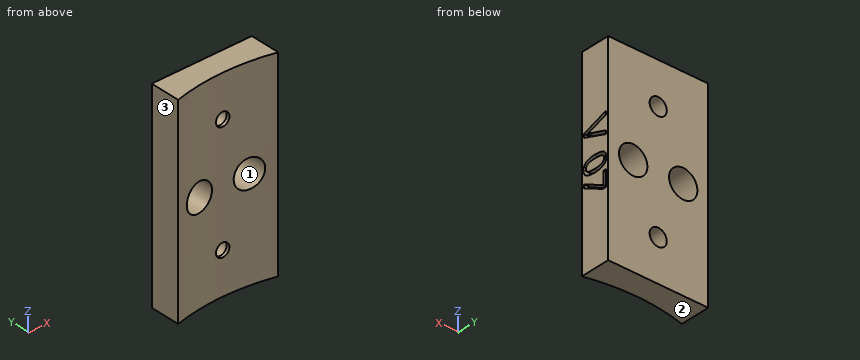
Autodesk Inventor part; units mm, degrees
ref_plane "YZ Plane" through (0, 0, 0) normal (1, 0, 0) x (0, 1, 0)
ref_plane "XZ Plane" through (0, 0, 0) normal (0, 1, 0) x (-1, 0, 0)
ref_plane "XY Plane" through (0, 0, 0) normal (0, 0, 1) x (1, 0, 0)
sketch "Sketch1" plane through (0, 0, 0) normal (0, 0, 1) x (1, 0, 0)
  arc A0 (19.05, 73.7803) -> (-19.05, 73.7803) centre (0, 0) ccw
  line L0 (0, 85.2103) -> (19.05, 85.2103)
  line L1 (19.05, 85.2103) -> (19.05, 73.7803)
  line L2 (0, 76.2) -> (0, 85.2103) construction
  line L3 (0, 85.2103) -> (-19.05, 85.2103)
  line L4 (-19.05, 85.2103) -> (-19.05, 73.7803)
  dimension "d0" = 152.4
  dimension "d1" = 19.05
  dimension "d2" = 11.43
extrude "Extrusion1" add sketch "Sketch1" along normal mid plane 76.2
sketch "Sketch23" plane through (-19.05, 85.2103, 38.1) normal (0, 1, 0) x (1, 0, 0)
  line L0 (38.1, 0) -> (0, 0) construction
  line L1 (19.05, 0) -> (19.05, 76.2) construction
  line L2 (0, 76.2) -> (38.1, 76.2) construction
  point P0 (19.05, 38.1)
  point P1 (19.05, 15.875)
  point P2 (19.05, 60.325)
  dimension "d183" = 15.875
  dimension "d184" = 15.875
hole "Hole2" at (0, 85.2103, 22.225) at (0, 85.2103, -22.225) direction (0, -1, 0) diameter 5.1054 end through all counterbore diameter 6.5278 counterbore depth 7.874
sketch "Sketch24" plane through (-19.05, 85.2103, 38.1) normal (0, 1, 0) x (1, 0, 0)
  line L0 (0, 76.2) -> (0, 0) construction
  line L1 (0, 38.1) -> (38.1, 38.1) construction
  line L2 (38.1, 76.2) -> (38.1, 0) construction
  line L3 (38.1, 0) -> (0, 0) construction
  line L4 (19.05, 0) -> (19.05, 76.2) construction
  line L5 (0, 76.2) -> (38.1, 76.2) construction
  line L6 (28.575, 38.1) -> (28.575, 38.1) construction
  line L7 (33.9725, 38.1) -> (33.9725, 38.1)
  line L8 (23.1775, 38.1) -> (23.1775, 38.1)
  arc A0 (23.1775, 38.1) -> (33.9725, 38.1) centre (28.575, 38.1) ccw
  arc A1 (33.9725, 38.1) -> (23.1775, 38.1) centre (28.575, 38.1) ccw
  line L9 (9.525, 38.1) -> (9.525, 38.1) construction
  line L10 (14.9225, 38.1) -> (14.9225, 38.1)
  line L11 (4.1275, 38.1) -> (4.1275, 38.1)
  arc A2 (4.1275, 38.1) -> (14.9225, 38.1) centre (9.525, 38.1) ccw
  arc A3 (14.9225, 38.1) -> (4.1275, 38.1) centre (9.525, 38.1) ccw
  point P0 (19.05, 38.1)
  point P1 (28.575, 38.1)
  point P2 (9.525, 38.1)
  dimension "d192" = 9.525
  dimension "d194" = 9.525
  dimension "d195" = 19.05
  dimension "d199" = 10.795
  dimension "d200" = 10.795
extrude "Extrusion8" cut sketch "Sketch24" against normal through all
sketch "Sketch25" plane through (19.05, 73.7803, 38.1) normal (1, 0, 0) x (0, 0, -1)
  line L0 (0, 11.43) -> (0, 0) construction
  line L1 (0, 5.715) -> (76.2, 5.715) construction
  line L2 (76.2, 11.43) -> (76.2, 0) construction
  line L3 (32.8705, 10.4775) -> (29.59, 0.9525)
  line L4 (29.59, 0.9525) -> (28.2238, 0.9525)
  line L5 (28.2238, 0.9525) -> (24.9433, 10.4775)
  line L6 (24.9433, 10.4775) -> (26.3018, 10.4775)
  line L7 (26.3018, 10.4775) -> (28.9416, 2.5657)
  line L8 (28.9416, 2.5657) -> (31.5815, 10.4775)
  line L9 (31.5815, 10.4775) -> (32.8705, 10.4775)
  spline S0 degree 2 poles (43.6382, 5.715) (43.6382, 3.1524) (42.1485, 0.7518) (40.597, 0.7518) knots 0 0 0 1 2 2 2
  spline S1 degree 2 poles (40.597, 0.7518) (39.0224, 0.7518) (37.5481, 3.1987) (37.5481, 5.7073) knots 0 0 0 1 2 2 2
  spline S2 degree 2 poles (37.5481, 5.7073) (37.5481, 8.2854) (39.0378, 10.6705) (40.597, 10.6705) knots 0 0 0 1 2 2 2
  spline S3 degree 2 poles (40.597, 10.6705) (42.1639, 10.6705) (43.6382, 8.2005) (43.6382, 5.715) knots 0 0 0 1 2 2 2
  spline S4 degree 2 poles (42.0019, 2.8127) (42.1871, 3.2836) (42.3415, 4.7347) (42.3415, 5.715) knots 0 0 0 1 2 2 2
  spline S5 degree 2 poles (42.3415, 5.715) (42.3415, 6.6953) (42.1871, 8.1387) (41.9941, 8.625) knots 0 0 0 1 2 2 2
  spline S6 degree 2 poles (41.9941, 8.625) (41.8012, 9.1113) (41.1296, 9.613) (40.597, 9.613) knots 0 0 0 1 2 2 2
  spline S7 degree 2 poles (40.597, 9.613) (40.0644, 9.613) (39.3775, 9.1113) (39.1768, 8.6096) knots 0 0 0 1 2 2 2
  spline S8 degree 2 poles (39.1768, 8.6096) (38.9838, 8.1233) (38.8449, 6.6413) (38.8449, 5.7073) knots 0 0 0 1 2 2 2
  spline S9 degree 2 poles (38.8449, 5.7073) (38.8449, 4.7038) (38.9684, 3.3608) (39.1691, 2.8359) knots 0 0 0 1 2 2 2
  spline S10 degree 2 poles (39.1691, 2.8359) (39.3543, 2.3419) (40.0413, 1.8093) (40.597, 1.8093) knots 0 0 0 1 2 2 2
  spline S11 degree 2 poles (40.597, 1.8093) (41.1219, 1.8093) (41.8089, 2.311) (42.0019, 2.8127) knots 0 0 0 1 2 2 2
  line L10 (50.8399, 9.0495) -> (46.718, 0.9525)
  line L11 (46.718, 0.9525) -> (45.3595, 0.9525)
  line L12 (45.3595, 0.9525) -> (49.7129, 9.3583)
  line L13 (49.7129, 9.3583) -> (44.7961, 9.3583)
  line L14 (44.7961, 9.3583) -> (44.7961, 10.4775)
  line L15 (44.7961, 10.4775) -> (50.8399, 10.4775)
  line L16 (50.8399, 10.4775) -> (50.8399, 9.0495)
  point P0 (38.1, -73.7803)
extrude "Extrusion9" cut sketch "Sketch25" against normal blind 2.54
equation "\"d51\" = 0.125 * Sketch8_Pitch"
equation "\"Sketch8_Pitch\" = 0.79375"
equation "\"d53\" = 60deg"
equation "\"d72\" = 0.125 * Sketch10_Pitch"
equation "\"Sketch10_Pitch\" = 0.79375"
equation "\"d74\" = 60deg"
equation "\"d93\" = 0.125 * Sketch12_Pitch"
equation "\"Sketch12_Pitch\" = 0.79375"
equation "\"d95\" = 60deg"
equation "\"d114\" = 0.125 * Sketch14_Pitch"
equation "\"Sketch14_Pitch\" = 0.79375"
equation "\"d116\" = 60deg"
equation "\"d135\" = 0.125 * Sketch16_Pitch"
equation "\"Sketch16_Pitch\" = 0.79375"
equation "\"d137\" = 60deg"
equation "\"d156\" = 0.125 * Sketch18_Pitch"
equation "\"Sketch18_Pitch\" = 0.79375"
equation "\"d158\" = 60deg"
properties part number "finderSupportPartV07" material "PC/ABS Plastic"
Geometry: final body of the model. Coordinates: model frame, mm. Face numbers are marked on the shaded views. Give positions to 0.01 mm unless a question says otherwise; leave off trailing zeros. Loops run counter-clockwise (first coordinate to the right, second up) from the corner with the lowest first, then second, coordinate; pieces in that order, holes last. Notation, with made-up numbers: (-16, 86.5) -> (24, 86.5) arc R23 cw to (24, 99.5) -> close; hole circle Ø1 at (67, 29.25). An arc over 180 degrees is marked (long way). Put each result on its own line as item: value.
1. Pin query (flat end, axial travel): P1, Ø0.6, axis at x = 18, z = 6, coming from the -Y side; P2, Ø3.5, axis at x = -1.5, z = -23, coming from the +Y side; P3, Ø0.7, axis at x = 17.5, z = 12.5, coming from the -Y side; P4, Ø7.5, axis at x = 0, z = -22.225, coming from the -Y side. Return the tip coordinate at first contact, or that it passes through.
Taken from the geometry:
P1: stops at y = 73.97
P2: stops at y = 85.21
P3: stops at y = 74.08
P4: stops at y = 76.11
2. Cut plane B-B (z = -20.5). Return the cut outline in (x, y), plus the area to 3 significant figures.
Taken from the geometry:
outline: (-19.05, 73.78) arc R76.2 cw to (-1.88, 76.18) -> (-1.88, 77.34) -> (-2.77, 77.34) -> (-2.77, 85.21) -> (-19.05, 85.21) -> close; (1.88, 76.18) arc R76.2 cw to (19.05, 73.78) -> (19.05, 85.21) -> (2.77, 85.21) -> (2.77, 77.34) -> (1.88, 77.34) -> close
area: 326 mm2
3. Ray query, line 1 along Z through (x, y) = (0, 79.25); line 2 along X through (y, z) = (82.25, 0); line 3 along Z through (x, y) = (0, 77.05). Return the intervals inside material, ascending. Write a range as [from, to].
Taken from the geometry:
line 1: z = [-38.1, -25.49], [-18.96, 18.96], [25.49, 38.1]
line 2: x = [-19.05, -14.92], [-4.13, 4.13], [14.92, 16.51]
line 3: z = [-38.1, -24.78], [-19.67, 19.67], [24.78, 38.1]
4. Pull-direction query (X, two-part tool) for the marked faces 1, 2 and 3; classes: released by +X, released by -X, zero draft, split by the parting line, or undercut.
Taken from the geometry:
face 1: undercut
face 2: zero draft
face 3: released by -X
5. Cut plane C-C (z = 4). Return the cut outline in (x, y).
Taken from the geometry:
outline: (-19.05, 73.78) arc R76.2 cw to (-13.15, 75.06) -> (-13.15, 85.21) -> (-19.05, 85.21) -> close; (-5.9, 75.97) arc R76.2 cw to (5.9, 75.97) -> (5.9, 85.21) -> (-5.9, 85.21) -> close; (13.15, 75.06) arc R76.2 cw to (19.05, 73.78) -> (19.05, 85.21) -> (13.15, 85.21) -> close
6. Cut plane A-A (x = 0). Return the cut outline in (y, z).
Taken from the geometry:
outline: (76.2, -38.1) -> (85.21, -38.1) -> (85.21, -25.49) -> (77.34, -25.49) -> (77.34, -24.78) -> (76.2, -24.78) -> close; (76.2, -19.67) -> (77.34, -19.67) -> (77.34, -18.96) -> (85.21, -18.96) -> (85.21, 18.96) -> (77.34, 18.96) -> (77.34, 19.67) -> (76.2, 19.67) -> close; (76.2, 24.78) -> (77.34, 24.78) -> (77.34, 25.49) -> (85.21, 25.49) -> (85.21, 38.1) -> (76.2, 38.1) -> close
7. Cut plane D-D (x = 6). Return the cut outline in (y, z), plus the area to 3 significant figures.
Taken from the geometry:
outline: (75.96, -38.1) -> (85.21, -38.1) -> (85.21, -4.09) -> (75.96, -4.09) -> close; (75.96, 4.09) -> (85.21, 4.09) -> (85.21, 38.1) -> (75.96, 38.1) -> close
area: 629 mm2
